Input: part model. Units: mm. Frame: model coordinates. A direction names the side the tool comes from. Give positions to 0.01 mm unless a question says otherwise; leave off trailing zeros. Order: outer loops, then holes, each group sorted by start corner. A loop starts at its lowest first (then second) coordinate and runs counter-clockwise, first axis right, second up. Notation, with made-up numbers: (66.5, 3.5) - (116.5, 3.5) arc R13 cw to (116.5, 19.5) - close; hole circle Ø6 at (61.25, 61). An arc over 180 degrees is marked (long way). Answer in a Markdown table with one row per item. Add a question column.
1. Ray query, line 1 (Z direction, x = 0, y = 2.55); line 2 (X direction, y = 2.3, z = -5.1); line 3 (Z direction, x = -0.5, y = 1.75). Return the intervals inside material, ascending. Write a range as [from, to].
2. Section query B-B on y = 4.5. Count the separate pieces of the cut face and the enclosed holes in it, and give its area (3 significant figures).
3. Contact query for flat-ended pins moving along their axis: pin 1 (1.2 mm diameter, centred on x = 0, z = -22.9, fed in from +Y); pin 2 (2 mm diameter, centred on x = 3, y = 1, fed in from -Z); pin 3 (1.8 mm diameter, centred on x = 1, y = 2, fed in from +Z). Output: stop coordinate, or through.
4. Section query A-A on x = 0. Return loops of the section in (y, z), and give its area (3 significant figures).
5. Access query for faces 1 (the face through (-5, 3, 14)), 2 (the face through (-0.13, 2.91, -23.89)). Directions: +Z, -Z, +X, -X, +Y, -Y. A direction counts if a zero-diameter tool reaches every point of the face in a straight line with its end or side. Return the directions, or none.
6. Section query C-C on x = -10.5. Return loops of the section in (y, z).
7. Section query D-D on z = -22.9. Return loops of the section in (x, y).
8. Mould query, pull axis X, two halves, no side actions, for faces 3 (the face through (17.5, 3, 3)), 4 (the face through (-0.26, 2.909, -10.517)), 5 (the face through (-0.217, 2.909, -1.124)), 6 (the face through (0, 0, -7)). Classes: released by +X, released by -X, zero draft, split by the parting line, or undercut.
```python
from build123d import *

# Parameters (mm, degrees)
SKETCH1_R           = 1
BOSS_EXTRUDE1_DEPTH = 5.9
SKETCH2_W           = 10
SKETCH2_H           = 11.8
CUT_EXTRUDE1_DEPTH  = 10
SKETCH3_W           = 12.5
SKETCH3_H           = 5.9
BOSS_EXTRUDE2_DEPTH = 5
CUT_EXTRUDE2_REACH  = 7.9
SKETCH4_R           = 2.05


with BuildPart() as part:
    # Sketch1 → Boss-Extrude1 (new body)
    with BuildSketch(Plane(origin=(0, 0, 0), x_dir=(1, 0, 0), z_dir=(0, 1, 0))):
        with BuildLine():
            ThreePointArc((9.4, 12.5), (10.4, 13.5), (11.4, 12.5))
            Line((11.4, 12.5), (17.5, 12.5))
            ThreePointArc((17.5, 12.5), (0, 30), (-17.5, 12.5))
            Line((-17.5, 12.5), (-11.4, 12.5))
            ThreePointArc((-11.4, 12.5), (-10.4, 13.5), (-9.4, 12.5))
            Line((-9.4, 12.5), (-8.4, 12.5))
            ThreePointArc((-8.4, 12.5), (-7.4, 13.5), (-6.4, 12.5))
            Line((-6.4, 12.5), (-2, 12.5))
            ThreePointArc((-2, 12.5), (0, 14.5), (2, 12.5))
            Line((2, 12.5), (6.4, 12.5))
            ThreePointArc((6.4, 12.5), (7.4, 13.5), (8.4, 12.5))
            Line((8.4, 12.5), (9.4, 12.5))
        make_face()
        with Locations((0, 19.9)):
            Circle(SKETCH1_R, mode=Mode.SUBTRACT)
        with Locations((0, 22.9)):
            Circle(SKETCH1_R, mode=Mode.SUBTRACT)
        with BuildLine():
            Line((17.5, 12.5), (11.4, 12.5))
            ThreePointArc((11.4, 12.5), (10.4, 11.5), (9.4, 12.5))
            Line((9.4, 12.5), (8.4, 12.5))
            ThreePointArc((8.4, 12.5), (7.4, 11.5), (6.4, 12.5))
            Line((6.4, 12.5), (2, 12.5))
            ThreePointArc((2, 12.5), (0, 10.5), (-2, 12.5))
            Line((-2, 12.5), (-6.4, 12.5))
            ThreePointArc((-6.4, 12.5), (-7.4, 11.5), (-8.4, 12.5))
            Line((-8.4, 12.5), (-9.4, 12.5))
            ThreePointArc((-9.4, 12.5), (-10.4, 11.5), (-11.4, 12.5))
            Line((-11.4, 12.5), (-17.5, 12.5))
            ThreePointArc((-17.5, 12.5), (0, -5), (17.5, 12.5))
        make_face()
        with Locations((0, 2.1)):
            Circle(SKETCH1_R, mode=Mode.SUBTRACT)
        with Locations((0, 5.1)):
            Circle(SKETCH1_R, mode=Mode.SUBTRACT)
        with BuildLine():
            Line((17.5, -12.5), (17.5, 12.5))
            ThreePointArc((17.5, 12.5), (0, -5), (-17.5, 12.5))
            Line((-17.5, 12.5), (-17.5, -12.5))
            Line((-17.5, -12.5), (17.5, -12.5))
        make_face()
    extrude(amount=BOSS_EXTRUDE1_DEPTH)

    # Sketch2 → Cut-Extrude1 (cut)
    with BuildSketch(Plane(origin=(0, 5.9, 0), x_dir=(1, 0, 0), z_dir=(0, 1, 0))):
        with Locations((0, -13.5)):
            Rectangle(SKETCH2_W, SKETCH2_H)
    extrude(amount=-CUT_EXTRUDE1_DEPTH, mode=Mode.SUBTRACT)

    # Sketch3 → Boss-Extrude2 (add)
    with BuildSketch(Plane.XY.offset(12.5)):
        with Locations((-11.25, 2.95)):
            Rectangle(SKETCH3_W, SKETCH3_H)
        with Locations((11.25, 2.95)):
            Rectangle(SKETCH3_W, SKETCH3_H)
    extrude(amount=BOSS_EXTRUDE2_DEPTH)

    # Sketch4 → Cut-Extrude2 (cut, up to next)
    with BuildSketch(Plane(origin=(0, 5.9, 0), x_dir=(1, 0, 0), z_dir=(0, 1, 0)), mode=Mode.PRIVATE) as cut_extrude2_sk1:
        with Locations((-5, -7.6)):
            Circle(SKETCH4_R)
    cut_extrude2_tool1 = extrude(cut_extrude2_sk1.sketch, amount=-CUT_EXTRUDE2_REACH, mode=Mode.PRIVATE) & part.part
    add(cut_extrude2_tool1.solids().sort_by_distance((-5, 5.9, 7.6))[0], mode=Mode.SUBTRACT)
    # Sketch4 → Cut-Extrude2 (cut, up to next)
    with BuildSketch(Plane(origin=(0, 5.9, 0), x_dir=(1, 0, 0), z_dir=(0, 1, 0)), mode=Mode.PRIVATE) as cut_extrude2_sk2:
        with Locations((5, -7.6)):
            Circle(SKETCH4_R)
    cut_extrude2_tool2 = extrude(cut_extrude2_sk2.sketch, amount=-CUT_EXTRUDE2_REACH, mode=Mode.PRIVATE) & part.part
    add(cut_extrude2_tool2.solids().sort_by_distance((5, 5.9, 7.6))[0], mode=Mode.SUBTRACT)


solid = part.part
```
Answer:
| question | item | result |
|---|---|---|
| 1 | line 1 | z = [-30, -23.9], [-21.9, -20.9], [-18.9, -14.5], [-10.5, -6.1], [-4.1, -3.1], [-1.1, 7.6] |
| 1 | line 2 | x = [-17.5, -1], [1, 17.5] |
| 1 | line 3 | z = [-29.99, -23.77], [-22.03, -20.77], [-19.03, -14.44], [-10.56, -5.97], [-4.23, -2.97], [-1.23, 7.6] |
| 2 | separate pieces | 1 |
| 2 | enclosed holes | 9 |
| 2 | area | 1,370 mm² |
| 3 | pin 1 | passes through |
| 3 | pin 2 | stops at z = -29.89 |
| 3 | pin 3 | stops at z = 7.6 |
| 4 | outline | (0, -30) - (5.9, -30) - (5.9, -23.9) - (0, -23.9) - close; (0, -21.9) - (5.9, -21.9) - (5.9, -20.9) - (0, -20.9) - close; (0, -18.9) - (5.9, -18.9) - (5.9, -14.5) - (0, -14.5) - close; (0, -10.5) - (5.9, -10.5) - (5.9, -6.1) - (0, -6.1) - close; (0, -4.1) - (5.9, -4.1) - (5.9, -3.1) - (0, -3.1) - close; (0, -1.1) - (5.9, -1.1) - (5.9, 7.6) - (0, 7.6) - close |
| 4 | area | 151 mm² |
| 5 | face 1 | +Z, +Y, -Y |
| 5 | face 2 | +Y, -Y |
| 6 | outline | (0, -26.5) - (5.9, -26.5) - (5.9, -13.49) - (0, -13.49) - close; (0, -11.51) - (5.9, -11.51) - (5.9, 17.5) - (0, 17.5) - close |
| 7 | outline | (-14.07, 0) - (-1, 0) - (-1, 5.9) - (-14.07, 5.9) - close; (1, 0) - (14.07, 0) - (14.07, 5.9) - (1, 5.9) - close |
| 8 | face 3 | released by +X |
| 8 | face 4 | undercut |
| 8 | face 5 | undercut |
| 8 | face 6 | zero draft |
